Check sheet for the modelled part. Datum: model origin and axes. Units: mm. A direction names the side the tool comes from. Coordinates: 2 decimals unless noted, no trailing zeros. Loops run counter-clockwise (first coordinate to the right, second up) from the corner with the lowest first, then second, coordinate; pieces in that order, holes last. Notation, with made-up numbers: (-7, 70) - (51, 70) arc R23 ccw to (51, 79) - close; hole circle Ø10 at (82, 13.5). An arc over 180 degrees is marked (long way). Use a Markdown table: item, result. Add a question column.
1) Sectioned sample at B-B, the plane z = 6. Enter the section's corners in (x, y), then the cut area to 3 significant figures.
2) Draft check along X on faces 1 (the flat face through (80, 10, 17)), 2 (the flat face through (68, 9.9, 13.5)). Enter one of: pulls with the +X half, pulls with the -X half, needs draft (parallel to the pull), parting line crosses it, or undercut.
3) Tool access check on faces 3 (the flat face through (-52, 9.9, 13.5)), 4 (the flat face through (80, 49, 17)). Record the directions out of +Z, -Z, +X, -X, +Y, -Y that give a thin tool (end or side, any length) a straight path to the whole face; none if there is none.
4) Sectioned sample at C-C, the plane z = 14.5. State how many separate pieces and enclosed holes the cut face has, then the cut area to 3 significant figures.
5) Thickness scan on line 1 (Y direction, x = 15, z = 2); line 2 (X direction, y = 30, z = 2.5); line 3 (X direction, y = 36, z = 14). Record the ranges inside material, lowest first.
6) Go/stop test with flat-tipped pins: P1, Ø5.5, axis at x = 55, y = 13.5, coming from the +Z side; P2, Ø4, axis at x = 7, y = 6, coming from the +Z side; P3, Ø2.5, axis at x = -39, y = 46.5, coming from the +Z side. Record where each tip stops, or that it passes through.
7) Sectioned sample at A-A, the plane y = 30. Enter the section's corners in (x, z), then the cut area to 3 significant figures.
from build123d import *

# Parameters (mm, degrees)
BOSS_EXTRUDE1_DEPTH = 60
CUT_EXTRUDE1_DEPTH  = 30


with BuildPart() as part:
    # Sketch1 → Boss-Extrude1 (new body)
    with BuildSketch(Plane(origin=(0, 0, 0), x_dir=(1, 0, 0), z_dir=(0, 1, 0))):
        Polygon((-98.5, 0), (98.5, 0), (98.5, -17), (93.5, -17), (90.5, -10), (85.5, -10), (82.5, -17), (77.5, -17), (74.5, -10), (69.5, -10), (66.5, -17), (61.5, -17), (58.5, -10), (53.5, -10), (50.5, -17), (45.5, -17), (42.5, -10), (37.5, -10), (34.5, -17), (29.5, -17), (26.5, -10), (21.5, -10), (18.5, -17), (13.5, -17), (10.5, -10), (5.5, -10), (2.5, -17), (-2.5, -17), (-5.5, -10), (-10.5, -10), (-13.5, -17), (-18.5, -17), (-21.5, -10), (-26.5, -10), (-29.5, -17), (-34.5, -17), (-37.5, -10), (-42.5, -10), (-45.5, -17), (-50.5, -17), (-53.5, -10), (-58.5, -10), (-61.5, -17), (-66.5, -17), (-69.5, -10), (-74.5, -10), (-77.5, -17), (-82.5, -17), (-85.5, -10), (-90.5, -10), (-93.5, -17), (-98.5, -17), align=None)
    extrude(amount=BOSS_EXTRUDE1_DEPTH)

    # Sketch2 → Cut-Extrude1 (cut, symmetric)
    with BuildSketch(Plane.XY):
        with BuildLine():
            Line((-78.5, 40), (78.5, 40))
            ThreePointArc((78.5, 40), (88.5, 30), (78.5, 20))
            Line((78.5, 20), (-78.5, 20))
            ThreePointArc((-78.5, 20), (-88.5, 30), (-78.5, 40))
        make_face()
    extrude(amount=CUT_EXTRUDE1_DEPTH, both=True, mode=Mode.SUBTRACT)


solid = part.part
Solved:
| question | item | result |
|---|---|---|
| 1 | outline | (-98.5, 0) - (98.5, 0) - (98.5, 60) - (-98.5, 60) - close; hole (-78.5, 20) - (78.5, 20) arc R10 ccw to (78.5, 40) - (-78.5, 40) arc R10 ccw to start |
| 1 | area | 8,370 mm2 |
| 2 | face 1 | needs draft |
| 2 | face 2 | undercut |
| 3 | face 3 | +Z, +Y, -Y |
| 3 | face 4 | +Z, +X, -X, +Y, -Y |
| 4 | separate pieces | 24 |
| 4 | enclosed holes | 0 |
| 4 | area | 3,880 mm2 |
| 5 | line 1 | y = 0 to 20, 40 to 60 |
| 5 | line 2 | x = -98.5 to -88.5, 88.5 to 98.5 |
| 5 | line 3 | x = -98.5 to -92.21, 92.21 to 98.5 |
| 6 | P1 | stops at z = 12.92 |
| 6 | P2 | stops at z = 11.17 |
| 6 | P3 | stops at z = 10 |
| 7 | outline | (-98.5, 0) - (-88.5, 0) - (-88.5, 10) - (-90.5, 10) - (-93.5, 17) - (-98.5, 17) - close; (88.5, 0) - (98.5, 0) - (98.5, 17) - (93.5, 17) - (90.5, 10) - (88.5, 10) - close |
| 7 | area | 291 mm2 |
